Answer from the drawing. Dimensions are ordinates in mm from the lowest x, y and z of the part. A direction names the side the tool comes from. Round coordinates to 2 decimals unless told otherwise and drop trailing zeros. Loops run counter-clockwise (first coordinate to the right, second up) from the corner with the lowest first, then second, coordinate; pieces in that order, holes last. Notation, with made-up numbers: M 69.25,-12 L 119.25,-12 A22 cw 119.25,0 Z; hole C 30.25,64.25 d5. An arc over 180 degrees is marked long. Write each question's results on one line, items separated by ' | '.
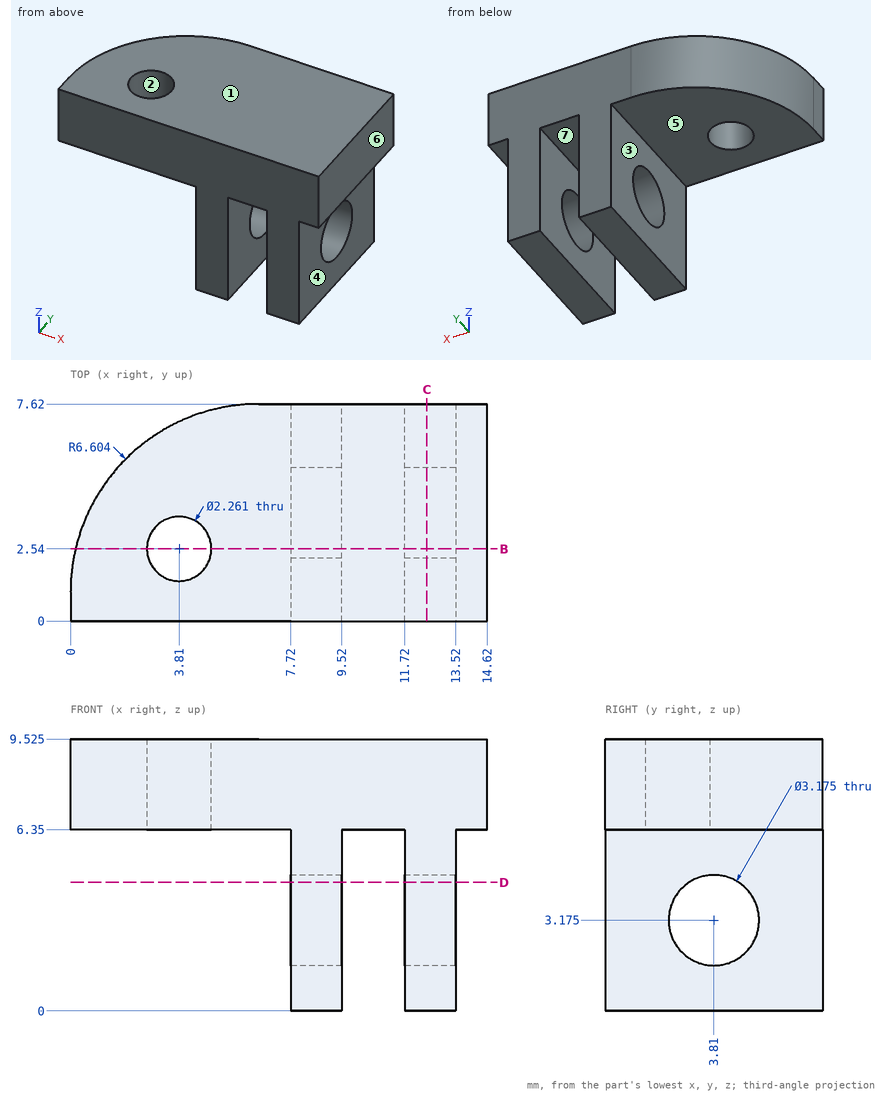
1. Find the intervals of material crossed by L1, parallel to X at y = 1, z = 6; L2, parallel to Y at x = 3.81, z = 8.4; L3, parallel to X at y = 1.75, z = 6.5, in increasing order.
Completed:
L1: x = 7.72 to 9.52, 11.72 to 13.52 | L2: y = 0 to 1.41, 3.67 to 7 | L3: x = 0.04 to 3, 4.62 to 14.62
2. Find section D-D, the plane z = 4.5. Give the vertices of the cut face in (x, y) (1 decimal).
Completed:
outline: M 7.7,0 L 9.5,0 L 9.5,2.9 L 7.7,2.9 Z; M 7.7,4.7 L 9.5,4.7 L 9.5,7.6 L 7.7,7.6 Z; M 11.7,0 L 13.5,0 L 13.5,2.9 L 11.7,2.9 Z; M 11.7,4.7 L 13.5,4.7 L 13.5,7.6 L 11.7,7.6 Z
3. Find section C-C, the plane x = 12.5. Give the vertices of the cut face in (y, z) (1 decimal).
Completed:
outline: M 0,0 L 7.6,0 L 7.6,9.5 L 0,9.5 Z; hole C 3.8,3.2 d3.2
4. Given P1, Ø3, axis at y = 4, z = 4.5, coming from the -X side; P2, Ø0.9, axis at x = 14.5, y = 5.5, coming from the -Z side, each flat-ended and moving along its own axis, determine where each tip first touches the part or whether it passes through.
Completed:
P1: stops at x = 7.72 | P2: stops at z = 6.35
5. Determine the mould class of the marked faces 1, 2, 3 and 4 for opening direction X: released by +X, released by -X, zero draft, split by the parting line, or undercut.
Completed:
face 1: zero draft | face 2: undercut | face 3: released by -X | face 4: released by +X
6. Find section B-B, the plane y = 2.54. Count the separate pieces of the cut face and the enclosed holes in it.
Completed:
separate pieces: 4 | enclosed holes: 0
7. Which of the six approach directions +Z, -Z, +X, -X, +Y, -Y give full straight-line access (tool end or side, diameter ignored) to the marked faces 5, 6 and 7?
Completed:
face 5: -Z, -X, +Y, -Y | face 6: +Z, -Z, +X, +Y, -Y | face 7: -Z, +Y, -Y
